```python
from build123d import *

# Parameters (mm, degrees)
SKETCH1_W           = 12
SKETCH1_H           = 18.25
SKETCH2_R           = 3.7145
CUT_EXTRUDE1_DEPTH  = 8.5725
SKETCH3_W           = 87
SKETCH3_H           = 124
BOSS_EXTRUDE1_DEPTH = 8
FILLET1_R           = 4
SKETCH6_R           = 13.15
CUT_EXTRUDE2_DEPTH  = 12
SKETCH12_R          = 4.075
CUT_EXTRUDE6_DEPTH  = 2.56
SKETCH12_6_R        = 2.5
CUT_EXTRUDE7_DEPTH  = 8
FILLET2_R           = 0.5
SKETCH15_W          = 5
SKETCH15_H          = 124
BOSS_EXTRUDE2_DEPTH = 15


with BuildPart() as part:
    # Sketch1 → Revolve1 (revolve)
    with BuildSketch(Plane.XY):
        with Locations((14.255, 9.125)):
            Rectangle(SKETCH1_W, SKETCH1_H)
    revolve(axis=Axis((8.255, 0, 0), (1, 0, 0)))

    # Sketch2 → Cut-Extrude1 (cut)
    with BuildSketch(Plane.ZY.offset(-8.255)):
        Circle(SKETCH2_R)
    extrude(amount=-CUT_EXTRUDE1_DEPTH, mode=Mode.SUBTRACT)

    # Sketch6 → Cut-Extrude2 (cut)
    with BuildSketch(Plane.ZY.offset(-8.255)):
        Circle(SKETCH6_R)
    extrude(amount=-CUT_EXTRUDE2_DEPTH, mode=Mode.SUBTRACT)


with BuildPart() as body_2:
    # Sketch3 → Boss-Extrude1 (new body)
    with BuildSketch(Plane(origin=(20.255, 0, 0), x_dir=(0, 0, -1), z_dir=(1, 0, 0))):
        Rectangle(SKETCH3_W, SKETCH3_H)
    extrude(amount=BOSS_EXTRUDE1_DEPTH)

    # Fillet1
    fillet1_edges = [body_2.edges().sort_by_distance(p)[0] for p in [
        (28.255, 0, -43.5),
        (28.255, 0, 43.5),
    ]]
    fillet(fillet1_edges, radius=FILLET1_R)

    # Sketch12 → Cut-Extrude6 (cut)
    with BuildSketch(Plane(origin=(28.255, 0, 0), x_dir=(0, 0, -1), z_dir=(1, 0, 0))):
        Circle(SKETCH12_R)
    extrude(amount=-CUT_EXTRUDE6_DEPTH, mode=Mode.SUBTRACT)

    # Sketch12<6> → Cut-Extrude7 (cut)
    with BuildSketch(Plane(origin=(28.255, 0, 0), x_dir=(0, 0, -1), z_dir=(1, 0, 0))):
        Circle(SKETCH12_6_R)
    extrude(amount=-CUT_EXTRUDE7_DEPTH, mode=Mode.SUBTRACT)

    # Fillet2
    fillet2_edges = [body_2.edges().sort_by_distance(p)[0] for p in [
        (28.255, 0, 4.075),
    ]]
    fillet(fillet2_edges, radius=FILLET2_R)


with BuildPart() as part_1:
    add(part.part)

    # Combine1: union body 2
    add(body_2.part)

    # Sketch15 → Boss-Extrude2 (add)
    with BuildSketch(Plane.ZY.offset(-20.255)):
        with Locations((-41, 0)):
            Rectangle(SKETCH15_W, SKETCH15_H)
        with Locations((41, 0)):
            Rectangle(SKETCH15_W, SKETCH15_H)
    extrude(amount=BOSS_EXTRUDE2_DEPTH)


solid = part_1.part
```
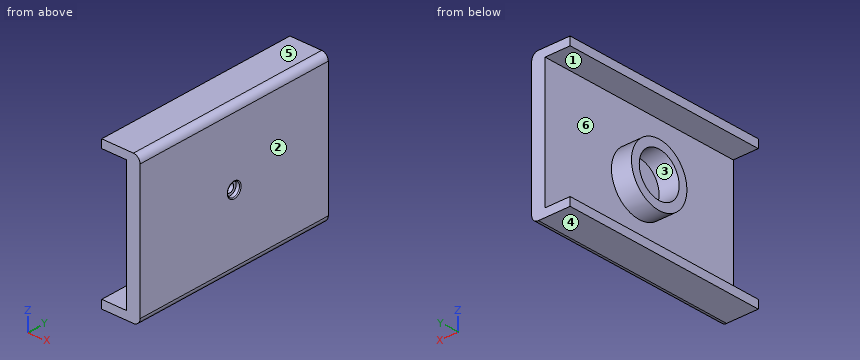
Verification items for the finished model (mm, model axes). Face numbers are marked on the shaded views. A direction names the side the tool comes from. Round coordinates to 2 decimals unless told otherwise and drop trailing zeros. Loops run counter-clockwise (first coordinate to the right, second up) from the corner with the lowest first, then second, coordinate; pieces in that order, holes last. Notation, with made-up numbers: (-29.75, -9) -> (11.25, -9) arc R15 cw to (11.25, 4) -> close; hole circle Ø1 at (51.25, -8). An arc over 180 degrees is marked (long way). Answer as a JSON object with one key per item and string values.
Q1. Section check A-A (x = 11.75). Record the boundary of the cut face in (y, z), then the cut area to 3 significant figures.
Data:
{"outline": "(-62, -43.5) -> (62, -43.5) -> (62, -38.5) -> (-62, -38.5) -> close; (-62, 38.5) -> (62, 38.5) -> (62, 43.5) -> (-62, 43.5) -> close; circle Ø36.5 at (0, 0); hole circle Ø26.3 at (0, 0)", "area": "1,740 mm2"}
Q2. Section check C-C (y = 0). Record the boundary of the cut face in (x, z) (3 decimals), then the cut area to 3 significant figures.
Data:
{"outline": "(5.255, -43.5) -> (24.255, -43.5) arc R4 ccw to (28.255, -39.5) -> (28.255, -4.575) arc R0.5 ccw to (27.755, -4.075) -> (25.695, -4.075) -> (25.695, -2.5) -> (20.255, -2.5) -> (20.255, -13.15) -> (8.255, -13.15) -> (8.255, -18.25) -> (20.255, -18.25) -> (20.255, -38.5) -> (5.255, -38.5) -> close; (5.255, 38.5) -> (20.255, 38.5) -> (20.255, 18.25) -> (8.255, 18.25) -> (8.255, 13.15) -> (20.255, 13.15) -> (20.255, 2.5) -> (25.695, 2.5) -> (25.695, 4.075) -> (27.755, 4.075) arc R0.5 ccw to (28.255, 4.575) -> (28.255, 39.5) arc R4 ccw to (24.255, 43.5) -> (5.255, 43.5) -> close", "area": "913 mm2"}
Q3. Scan lines: line 1 (Y direction, x = 21.95, z = 0); line 2 (Y direction, x = 27.35, z = 0) (3 decimals); line 3 (Z direction, x = 14.25, y = -12). Record each from-to range of solid material in increasing order. Write a range as from..to.
Data:
{"line 1": "y = -62..-2.5, 2.5..62", "line 2": "y = -62..-4.075, 4.075..62", "line 3": "z = -43.5..-38.5, -13.75..-5.38, 5.38..13.75, 38.5..43.5"}
Q4. Go/stop test with flat-tipped pins: P1, Ø9, axis at y = -1, z = -0.5, coming from the +X side (3 decimals); P2, Ø6.5, axis at y = 0, z = 0, coming from the -X side (3 decimals); P3, Ø6.5, axis at y = 0, z = 0, coming from the +X side (3 decimals); P4, Ø1, axis at x = 9.5, z = -19.5, coming from the +Y side. Record where each tip stops, or that it passes through.
Data:
{"P1": "stops at x = 28.255", "P2": "stops at x = 20.255", "P3": "stops at x = 25.695", "P4": "passes through"}
Q5. Access from +Z, -Z, +X, -X, +Y, -Y to the whole of each face (thin tool, end or side, straight path). Record for the marked faces 1, 2 and 3.
Data:
{"face 1": "-X, +Y, -Y", "face 2": "+Z, -Z, +X, +Y, -Y", "face 3": "-X"}
Q6. Section check D-D (y = -31). Record the boundary of the cut face in (x, z) (3 decimals).
Data:
{"outline": "(5.255, -43.5) -> (24.255, -43.5) arc R4 ccw to (28.255, -39.5) -> (28.255, 39.5) arc R4 ccw to (24.255, 43.5) -> (5.255, 43.5) -> (5.255, 38.5) -> (20.255, 38.5) -> (20.255, -38.5) -> (5.255, -38.5) -> close"}
Q7. Draft check along Z on the marked faces 4, 5 and 6. Enter one of: pulls with the +Z half, pulls with the -Z half, needs draft (parallel to the pull), parting line crosses it, or undercut.
Data:
{"face 4": "pulls with the -Z half", "face 5": "pulls with the +Z half", "face 6": "undercut"}
Q8. Section check B-B (z = 0). Record the boundary of the cut face in (x, y) (3 decimals), then the cut area to 3 significant figures.
Data:
{"outline": "(8.255, -18.25) -> (20.255, -18.25) -> (20.255, -62) -> (28.255, -62) -> (28.255, -4.575) arc R0.5 ccw to (27.755, -4.075) -> (25.695, -4.075) -> (25.695, -2.5) -> (20.255, -2.5) -> (20.255, -13.15) -> (8.255, -13.15) -> close; (8.255, 13.15) -> (20.255, 13.15) -> (20.255, 2.5) -> (25.695, 2.5) -> (25.695, 4.075) -> (27.755, 4.075) arc R0.5 ccw to (28.255, 4.575) -> (28.255, 62) -> (20.255, 62) -> (20.255, 18.25) -> (8.255, 18.25) -> close", "area": "1,070 mm2"}
